Here's how the part is built. I have some questions about the finished solid (model axes, mm). Face numbers are marked on the shaded views. A direction names the side the tool comes from. Give positions to 0.01 mm unless a question says otherwise; leave off trailing zeros. Order: outer loops, then holes, each group sorted by start corner. A loop starts at its lowest first (then second) coordinate and runs counter-clockwise, first axis right, second up.
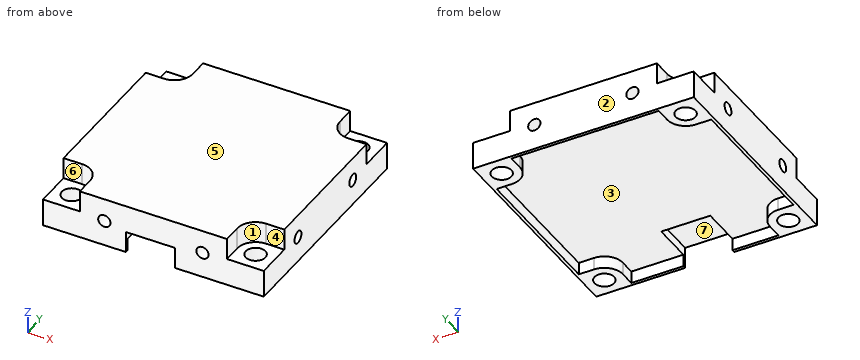
Autodesk Inventor part; units mm, degrees
ref_plane "Work Plane1" through (-18, 18, 0) normal (0.7071, 0.7071, 0) x (0, 0, 1)
ref_plane "YZ Plane" through (0, 0, 0) normal (1, 0, 0) x (0, 1, 0)
ref_plane "XZ Plane" through (0, 0, 0) normal (0, 1, 0) x (-1, 0, 0)
sketch "Sketch1" plane through (0, 0, 0) normal (0, 0, 1) x (1, 0, 0)
  line L0 (-21.6, 0) -> (3.6, 0) construction
  line L1 (0, -3.6) -> (0, 21.6) construction
  line L2 (-18, 18) -> (0, 18)
  line L3 (0, 18) -> (0, 0)
  line L4 (0, 0) -> (-18, 0)
  line L5 (-18, 0) -> (-18, 18)
  dimension "d0" = 18
  dimension "d1" = 18
extrude "Extrusion1" add sketch "Sketch1" along normal blind 8
sketch "Sketch2" plane through (0, 0, 8) normal (0, 0, 1) x (1, 0, 0)
  line L0 (-21.6, 0) -> (3.6, 0)
  line L1 (0, -3.6) -> (0, 21.6)
  point P0 (0, 0)
  point P1 (-15, 15)
  dimension "d4" = 15
  dimension "d5" = 15
hole "Hole1" at (-15, 15, 8) direction (0, 0, -1) diameter 3.2 end through all
sketch "Sketch3" plane through (0, 0, 8) normal (0, 0, 1) x (1, 0, 0)
  line L0 (-21.6, 0) -> (3.6, 0) construction
  line L1 (0, -3.6) -> (0, 21.6) construction
  line L2 (-18, 18) -> (-18, 0) construction
  line L3 (0, 18) -> (-18, 18) construction
  circle A0 centre (-15, 15) radius 1.6 construction
  arc A1 (-15, 12) -> (-12, 15) centre (-15, 15) ccw
  line L4 (-15, 12) -> (-18, 12)
  line L5 (-12, 15) -> (-12, 18)
  line L6 (-12, 18) -> (-18, 18)
  line L7 (-18, 12) -> (-18, 18)
  point P0 (0, 0)
  dimension "d13" = 3
extrude "Extrusion2" cut sketch "Sketch3" against normal blind 3.5
sketch "Sketch4" plane through (0, 0, 0) normal (0, 0, -1) x (-1, 0, 0)
  line L0 (21.6, 0) -> (-3.6, 0) construction
  line L1 (0, -3.6) -> (0, 21.6) construction
  line L2 (18, 18) -> (18, 0) construction
  line L3 (0, 18) -> (18, 18) construction
  line L4 (17.5, 0) -> (17.5, 12)
  circle A0 centre (15, 15) radius 1.6 construction
  line L5 (17.5, 12) -> (15, 12)
  arc A1 (12, 15) -> (15, 12) centre (15, 15) ccw
  line L6 (12, 15) -> (12, 17.5)
  line L7 (12, 17.5) -> (0, 17.5)
  line L8 (0, 17.5) -> (0, 0)
  line L9 (0, 0) -> (17.5, 0)
  dimension "d19" = 0.5
  dimension "d20" = 0.5
  dimension "d21" = 3
extrude "Extrusion3" cut sketch "Sketch4" against normal blind 2
sketch "Sketch5" plane through (-18, 18, 0) normal (0, 1, 0) x (1, 0, 0)
  line L0 (-3.6, 0) -> (21.6, 0)
  line L1 (18, 1.6) -> (18, -9.6)
  line L2 (18, -8) -> (6, -8)
  point P0 (18, 0)
  point P1 (10, -4.2)
  dimension "d24" = 8
  dimension "d25" = 3.8
hole "M3/6/10" at (-8, 18, 4.2) direction (0, -1, 0) diameter 2 depth 2
ref_plane "Work Plane1" through (-18, 18, 0) normal (0.7071, 0.7071, 0) x (0, 0, 1)
mirror "Mirror1" about plane through (-18, 18, 0) normal (0.7071, 0.7071, 0) of "M3/6/10"
pattern_circular "Circular Pattern1" count 4 over 360 about axis through (0, 0, -10) along (0, 0, 1)
sketch "Sketch7" plane through (0, 0, 0) normal (0, 0, -1) x (-1, 0, 0)
  line L0 (25.2, 0) -> (-25.2, 0) construction
  line L1 (0, -27.6) -> (0, 25.6) construction
  line L2 (18, -18) -> (-18, -18) construction
  line L3 (4.5, -11) -> (-3.5, -11)
  line L4 (-3.5, -11) -> (-3.5, -20)
  line L5 (-3.5, -20) -> (4.5, -20)
  line L6 (4.5, -20) -> (4.5, -11)
  line L7 (0.5, -11) -> (0.5, -20) construction
  line L8 (-18, -18) -> (-18, 18)
  point P0 (0, 0)
  dimension "d33" = 9
  dimension "d34" = 8
  dimension "d35" = 2
  dimension "d36" = 18.5
extrude "Extrusion4" cut sketch "Sketch7" against normal blind 3.5
equation "\"d20\" = d19"
properties part number "P106" material "ABS Plastic"
Q1. If we section it at D-D on x = 0: List the corners of the cut face in (y, z) for me, plus the area to 4 significant figures.
Filled sheet:
outline: (-18, 3.5) - (-11, 3.5) - (-11, 2) - (17.5, 2) - (17.5, 0) - (18, 0) - (18, 8) - (-18, 8) - close
area: 206.5 mm2
Q2. If we section it at A-A on y = -8: List the corners of the cut face in (x, z) for me.
Filled sheet:
outline: (-18, 0) - (-17.5, 0) - (-17.5, 2) - (17.5, 2) - (17.5, 0) - (18, 0) - (18, 3.2) - (16, 3.2) - (16, 5.2) - (18, 5.2) - (18, 8) - (-18, 8) - (-18, 5.2) - (-16, 5.2) - (-16, 3.2) - (-18, 3.2) - close
Q3. If we section it at C-C on z = 7: List the corners of the cut face in (x, y) for me, plus the area to 3 significant figures.
Filled sheet:
outline: (-18, -12) - (-15, -12) arc R3 cw to (-12, -15) - (-12, -18) - (12, -18) - (12, -15) arc R3 cw to (15, -12) - (18, -12) - (18, 12) - (15, 12) arc R3 cw to (12, 15) - (12, 18) - (-12, 18) - (-12, 15) arc R3 cw to (-15, 12) - (-18, 12) - close
area: 1,160 mm2
Q4. For the marked faces 4, 5, 6 and 7, which set-ups out of +Z, -Z, +X, -X, +Y, -Y let a thin tool reach every point of the face, with its end or its side?
Filled sheet:
face 4: +Z, +X, -Y
face 5: +Z, +X, -X, +Y, -Y
face 6: +Z, -X, -Y
face 7: -Z, -Y
Q5. Thinking about a two-plate mould opening in X: for the marked faces 1, 2 and 3, which applies, released by +X, released by -X, zero draft, split by the parting line, or undercut?
Filled sheet:
face 1: released by +X
face 2: zero draft
face 3: undercut
Q6. If we section it at B-B on x = -10.5: List the corners of the cut face in (y, z) for me, plus the area to 3 significant figures.
Filled sheet:
outline: (-18, 0) - (-17.5, 0) - (-17.5, 2) - (17.5, 2) - (17.5, 0) - (18, 0) - (18, 8) - (-18, 8) - close
area: 218 mm2
Q7. I need wall thicknesses on L1, parallel to X at y = -15, z = 2.15; L2, parallel to Y at x = -17.1, z = 4.2; L3, parallel to X at y = -15, z = 1.75. Which ranges of each line are inside material? Lowest first, please.
Filled sheet:
L1: x = -18 to -16.6, -13.4 to -4.5, 3.5 to 13.4, 16.6 to 18
L2: y = -18 to -9, -7 to 7, 9 to 18
L3: x = -18 to -16.6, -13.4 to -12, 12 to 13.4, 16.6 to 18
Q8. I'm going to push flat-ended pins straight in: P1, Ø1, axis at x = 8, z = 4, coming from the +Y side; P2, Ø12, axis at x = -2.5, y = -7, coming from the -Z side; P3, Ø0.9, axis at x = -17, z = 6, coming from the +Y side. Where does each tip first touch, or does it pass through?
Filled sheet:
P1: stops at y = 16
P2: stops at z = 2
P3: stops at y = 12
